Source: CAD feature listing. Evaluate the final solid. Frame: model axes, mm. A direction names the side the tool comes from. Give positions to 0.01 mm unless a question says otherwise; leave off trailing zeros. Loops run counter-clockwise (first coordinate to the right, second up) from the corner with the lowest first, then second, coordinate; pieces in that order, holes last. Notation, with made-up numbers: (85.25, -31) -> (120.25, -31) arc R27 ccw to (120.25, 8) -> close; hole circle Ø9 at (50.25, -27). An arc over 180 degrees is marked (long way). Answer as a JSON object with one key per item and string values. Group by question number.
from build123d import *

# Parameters (mm, degrees)
F0_R     = 20
F1_DEPTH = 25
F2_R     = 2.5
F3_DEPTH = 50
F4_R     = 10
F5_DEPTH = 25
F6_R     = 20
F6_R_2   = 10
F7_DEPTH = 5


with BuildPart() as f1:
    # F0 (on Right) → F1 (new body, symmetric)
    with BuildSketch(Plane.YZ):
        Circle(F0_R)
    extrude(amount=F1_DEPTH, both=True)

    # F2 (on face) → F3 (join)
    with BuildSketch(Plane.YZ.offset(25)):
        with Locations((-5, 5)):
            Circle(F2_R)
        with Locations((5, 5)):
            Circle(F2_R)
        with Locations((5, -5)):
            Circle(F2_R)
        with Locations((-5, -5)):
            Circle(F2_R)
    extrude(amount=F3_DEPTH)

    # F4 (on face) → F5 (join)
    with BuildSketch(Plane(origin=(-25, 0, 0), x_dir=(0, -1, 0), z_dir=(-1, 0, 0))):
        Circle(F4_R)
    extrude(amount=F5_DEPTH)

    # F6 (on face) → F7 (join)
    with BuildSketch(Plane(origin=(-50, 0, 0), x_dir=(0, -1, 0), z_dir=(-1, 0, 0))):
        Circle(F6_R)
        Circle(F6_R_2, mode=Mode.SUBTRACT)
    extrude(amount=-F7_DEPTH)


solid = f1.part
(1) Section query D-D on y = 17. Return the cut outline in (x, z), plus the area to 3 significant figures.
(2) Section query B-B on z = 14. Return the cut outline in (x, y).
(3) First-contact query: pin 1 (6 mm diameter, centred on x = -10, y = -6.5, fed in from -Z); pin 2 (10 mm diameter, centred on x = -14.5, y = -7, fed in from +Z); pin 3 (12 mm diameter, centred on x = -23, z = 13.5, fed in from +Y). Flat tips, straight axial feed; report the tip coordinate or a pass-through.
(4) Material intervals for line 1 (X direction, y = 15, z = 12); line 2 (X direction, y = -2.5, z = 0.5); line 3 (Y direction, x = -0.5, z = -1), sorted ascending. Write a range as from..to.
(5) Access query for faces 1 (the face through (-47.535, 4.336, -19.524)), 2 (the face through (-45, 5, 9)), 3 (the face through (49.65, -2.615, -4.249)). Directions: +Z, -Z, +X, -X, +Y, -Y. A direction counts if a zero-diameter tool reaches every point of the face in a straight line with its end or side. Return the directions, or none.
(6) Mould query, pull axis X, two halves, no side actions, for faces 4 (the face through (75, -5, -5)), 5 (the face through (-50, 0, 0)), 6 (the face through (-25, -5, 9)), 7 (the face through (49.65, 7.385, -4.249)). Classes: pulls with the +X half, pulls with the -X half, needs draft (parallel to the pull), parting line crosses it, or undercut.
(7) Section query A-A on y = 0. Return the cut outline in (x, z), plus the area to 3 significant figures.
Result:
{
 "1": {"outline": "(-50, -10.54) -> (-45, -10.54) -> (-45, 10.54) -> (-50, 10.54) -> close; (-25, -10.54) -> (25, -10.54) -> (25, 10.54) -> (-25, 10.54) -> close", "area": "1,160 mm²"},
 "2": {"outline": "(-50, -14.28) -> (-45, -14.28) -> (-45, 14.28) -> (-50, 14.28) -> close; (-25, -14.28) -> (25, -14.28) -> (25, 14.28) -> (-25, 14.28) -> close"},
 "3": {"pin 1": "z = -19.69", "pin 2": "z = 19.9", "pin 3": "y = 18.54"},
 "4": {"line 1": "-50..-45, -25..25", "line 2": "-50..25", "line 3": "-19.97..19.97"},
 "5": {"face 1": "+X, -X", "face 2": "none", "face 3": "+X"},
 "6": {"face 4": "pulls with the +X half", "face 5": "pulls with the -X half", "face 6": "undercut", "face 7": "needs draft"},
 "7": {"outline": "(-50, -20) -> (-45, -20) -> (-45, -10) -> (-25, -10) -> (-25, -20) -> (25, -20) -> (25, 20) -> (-25, 20) -> (-25, 10) -> (-45, 10) -> (-45, 20) -> (-50, 20) -> close", "area": "2,600 mm²"}
}
